Check sheet for the modelled part. Datum: model origin and axes. Units: mm. Round coordinates to 2 decimals unless told otherwise and drop trailing zeros. Order: outer loops, then holes, each group sorted by start corner. A loop starts at its lowest first (then second) coordinate and runs counter-clockwise, first axis right, second up.
(1) Depth check by flat-ended pin: pin 1 (5 mm diameter, centred on y = 0, z = -20, fed in from +X); pin 2 (2 mm diameter, centred on x = -21.5, z = -4.5, fed in from +Y); pin 3 (5 mm diameter, centred on y = 14.14, z = -14.14, fed in from -X); pin 4 (4 mm diameter, centred on y = -14.14, z = 14.14, fed in from -X). Enter the tip coordinate at first touch or a pass-through.
(2) Thickness scan on probe 1 along Z at (x, y) = (-5.75, -16); probe 2 along Y at (x, z) = (-5.5, 13); probe 3 along Y at (x, z) = (-2.25, -14.5). Record the ranges inside material, lowest first.
(3) Sectioned sample at A-A, the plane x = -11.75. Count the separate pieces of the cut face and the enclosed holes in it, and give its area (3 significant figures).
(4) Mould release check, pull along Z, two halves, no side actions. Record for faces 1 (the flat face through (-18.5, 0, 0)), 2 (the cylindrical face through (-8.381, -26.846, 5.961)), 3 (the flat face through (-30, 12.5, 27.5)): released by +Z, released by -Z, zero draft, split by the parting line, or undercut.
(5) Sectioned sample at C-C, the plane x = -21. Enter the section's corners in (y, z), and give its area (3 significant figures).
Autodesk Inventor part; units mm, degrees
ref_plane "YZ Plane" through (0, 0, 0) normal (1, 0, 0) x (0, 1, 0)
ref_plane "XZ Plane" through (0, 0, 0) normal (0, 1, 0) x (-1, 0, 0)
ref_plane "XY Plane" through (0, 0, 0) normal (0, 0, 1) x (1, 0, 0)
sketch "草图3" plane through (0, 0, 0) normal (1, 0, 0) x (0, 1, 0)
  circle A0 centre (0, 0) radius 8 construction
  circle A1 centre (0, -8) radius 2.1
  line L0 (0, 0) -> (0, -8) construction
  circle A2 centre (8, 0) radius 2.1
  circle A3 centre (0, 8) radius 2.1
  circle A4 centre (-8, 0) radius 2.1
  circle A5 centre (0, 0) radius 42.5
  dimension "d21" = 16
  dimension "d22" = 4.2
  dimension "d25" = 360
  dimension "d27" = 85
extrude "拉伸3" add sketch "草图3" against normal blind 18.5
sketch "草图6" plane through (-18.5, 0, 0) normal (-1, 0, 0) x (0, 0, 1)
  circle A0 centre (0, 0) radius 30
  circle A1 centre (0, 0) radius 42.5
  dimension "d30" = 60
extrude "拉伸4" add sketch "草图6" along normal blind 11.5
chamfer "倒角1" distance 5 angle 45 1 edges at (-18.5, 0, -30)
sketch "草图7" plane through (0, 0, 0) normal (1, 0, 0) x (0, 0, -1)
  circle A0 centre (0, 0) radius 27.5
  circle A1 centre (0, 0) radius 42.5
  dimension "d36" = 55
extrude "拉伸5" cut sketch "草图7" against normal blind 19
chamfer "倒角2" distance 2 angle 45 1 edges at (-19, 0, 27.5)
sketch "草图8" plane through (0, 0, 0) normal (1, 0, 0) x (0, 0, -1)
  circle A0 centre (0, 0) radius 20 construction
  circle A1 centre (20, 0) radius 2.1
  line L0 (20, 0) -> (0, 0) construction
  line L1 (14.1421, 14.1421) -> (0, 0) construction
  circle A2 centre (14.1421, 14.1421) radius 2.1
  line L2 (0, 20) -> (0, 0) construction
  circle A3 centre (0, 20) radius 2.1
  line L3 (-14.1421, 14.1421) -> (0, 0) construction
  circle A4 centre (-14.1421, 14.1421) radius 2.1
  line L4 (-20, 0) -> (0, 0) construction
  circle A5 centre (-20, 0) radius 2.1
  line L5 (-14.1421, -14.1421) -> (0, 0) construction
  circle A6 centre (-14.1421, -14.1421) radius 2.1
  line L6 (0, -20) -> (0, 0) construction
  circle A7 centre (0, -20) radius 2.1
  line L7 (14.1421, -14.1421) -> (0, 0) construction
  circle A8 centre (14.1421, -14.1421) radius 2.1
  dimension "d42" = 40
  dimension "d43" = 4.2
  dimension "d46" = 360
extrude "拉伸6" cut sketch "草图8" against normal through all
chamfer "倒角4" distance 1 angle 45 2 edges at (-19, 0, -42.5) (-30, 0, -42.5)
properties part number "主动轮"
Derived:
1. pin 1: stops at x = 0
1. pin 2: stops at y = 42.36
1. pin 3: stops at x = -18.5
1. pin 4: passes through
2. probe 1: z = -22.37 to -15.12, -13.16 to 13.16, 15.12 to 22.37
2. probe 2: y = -24.23 to -15.9, -12.38 to 12.38, 15.9 to 24.23
2. probe 3: y = -23.37 to -16.21, -12.07 to 12.07, 16.21 to 23.37
3. separate pieces: 1
3. enclosed holes: 12
3. area: 2,210 mm2
4. face 1: undercut
4. face 2: split by the parting line
4. face 3: zero draft
5. outline: circle Ø85 at (0, 0); hole circle Ø55 at (0, 0)
5. area: 3,300 mm2
